Here's how the part is built. I have some questions about the finished solid (model axes, mm). Give positions to 0.01 mm unless a question says otherwise; leave off trailing zeros. Loops run counter-clockwise (first coordinate to the right, second up) from the corner with the lowest first, then second, coordinate; pieces in that order, holes last. Notation, with made-up numbers: (-17, 15.25) - (21, 15.25) arc R22 ccw to (21, 41.25) - close; hole circle Ø10 at (1, 25.5). An arc over 180 degrees is marked (long way). Use one line per item in the form item = value.
from build123d import *

# Parameters (mm, degrees)
SKETCH1_R           = 100
BOSS_EXTRUDE1_DEPTH = 30
SKETCH2_R           = 25
CUT_EXTRUDE2_DEPTH  = 40
SKETCH3_R           = 4
CUT_EXTRUDE3_DEPTH  = 40
CHAMFER1_SIZE       = 1
CHAMFER2_SIZE       = 1


with BuildPart() as part:
    # Sketch1 → Boss-Extrude1 (new body)
    with BuildSketch(Plane.XY):
        Circle(SKETCH1_R)
    extrude(amount=BOSS_EXTRUDE1_DEPTH)

    # Sketch2 → Cut-Extrude2 (cut)
    with BuildSketch(Plane.XY):
        Circle(SKETCH2_R)
    extrude(amount=CUT_EXTRUDE2_DEPTH, mode=Mode.SUBTRACT)

    # Sketch3 → Cut-Extrude3 (cut)
    with BuildSketch(Plane.XY.offset(30)):
        with Locations((56.568542495, 56.568542495)):
            Circle(SKETCH3_R)
        with Locations((-56.568542495, 56.568542495)):
            Circle(SKETCH3_R)
        with Locations((-56.568542495, -56.568542495)):
            Circle(SKETCH3_R)
        with Locations((56.568542495, -56.568542495)):
            Circle(SKETCH3_R)
    extrude(amount=-CUT_EXTRUDE3_DEPTH, mode=Mode.SUBTRACT)

    # Chamfer1
    chamfer1_edges = [part.edges().sort_by_distance(p)[0] for p in [
        (-100, 0, 0),
    ]]
    chamfer(chamfer1_edges, length=CHAMFER1_SIZE)

    # Chamfer2
    chamfer2_edges = [part.edges().sort_by_distance(p)[0] for p in [
        (-100, 0, 30),
    ]]
    chamfer(chamfer2_edges, length=CHAMFER2_SIZE)


solid = part.part
(1) If we section it at A-A (y = 0): List the corners of the cut face in (x, z) for me, plus the area to 3 significant figures.
Geometry says:
outline = (-100, 1) - (-99, 0) - (-25, 0) - (-25, 30) - (-99, 30) - (-100, 29) - close; (25, 0) - (99, 0) - (100, 1) - (100, 29) - (99, 30) - (25, 30) - close
area = 4,500 mm²
(2) For P1, Ø3, axis at y = 24, z = 8, coming from the -X side; P2, Ø12, axis at y = -27, z = 3.5, coming from the +X side; P3, Ø12, axis at x = 12.5, z = 5.5, coming from the -Y side, each with a flat end and sliding along its axis, tell me the tip position at first contact or that it passes through.
Geometry says:
P1 = -97.44
P2 = 97.77
P3 = -99.79
(3) If we section it at C-C (z = 22.25): List the corners of the cut face in (x, y) for me.
Geometry says:
outline = circle Ø200 at (0, 0); hole circle Ø8 at (-56.57, -56.57); hole circle Ø8 at (-56.57, 56.57); hole circle Ø50 at (0, 0); hole circle Ø8 at (56.57, -56.57); hole circle Ø8 at (56.57, 56.57)
(4) Thinking about a two-plate mould opening in X: for faces 1 (the cylindrical face through (23.846, 7.509, 14.79)), 2 (the flat face through (21, -21, 30)), 3 (the cylindrical face through (95.38, 30.04, 14.8)), which applies, pulls with the +X half, pulls with the -X half, needs draft (parallel to the pull), parting line crosses it, or undercut?
Geometry says:
face_1 = undercut
face_2 = needs draft
face_3 = parting line crosses it
(5) If I drill on probe 1 along Y at (x, z) = (0, 9.75); probe 2 along Y at (x, z) = (54.5, 25.5), over which ranges is the centre line in solid material (lowest first)?
Geometry says:
probe_1 = -100 to -25, 25 to 100
probe_2 = -83.84 to -59.99, -53.14 to 53.14, 59.99 to 83.84
